from build123d import *

# Parameters (mm, degrees)
SKETCH_1_R      = 1.6
SKETCH_1_W      = 108
SKETCH_1_H      = 67.317279836
EXTRUDE_1_DEPTH = 2
FILLET_1_R      = 3


with BuildPart() as part:
    # ｽｹｯﾁ1 → ﾎﾞｽ - 押し出し1 (new body)
    with BuildSketch(Plane(origin=(0, 0, 0), x_dir=(1, 0, 0), z_dir=(0, 1, 0))):
        Polygon((-61, 40.658639918), (-135.317279836, 40.658639918), (-135.317279836, 60.658639918), (-142.317279836, 60.658639918), (-142.317279836, 40.658639918), (-61, -40.658639918), (61, -40.658639918), (142.317279836, 40.658639918), (142.317279836, 60.658639918), (135.317279836, 60.658639918), (135.317279836, 40.658639918), (61, 40.658639918), align=None)
        with Locations(Location((-57.5, -37.158639918, 0), (0, 0, 270))):
            Circle(SKETCH_1_R, mode=Mode.SUBTRACT)
        with Locations(Location((57.5, -37.158639918, 0), (0, 0, 270))):
            Circle(SKETCH_1_R, mode=Mode.SUBTRACT)
        with Locations(Location((-131.746212025, 37.087572106, 0), (0, 0, 270))):
            Circle(SKETCH_1_R, mode=Mode.SUBTRACT)
        with Locations(Location((131.746212025, 37.087572106, 0), (0, 0, 270))):
            Circle(SKETCH_1_R, mode=Mode.SUBTRACT)
        with Locations(Location((20, -37.158639918, 0), (0, 0, 270))):
            Circle(SKETCH_1_R, mode=Mode.SUBTRACT)
        with Locations(Location((-20, -37.158639918, 0), (0, 0, 270))):
            Circle(SKETCH_1_R, mode=Mode.SUBTRACT)
        with Locations(Location((20, 37.158639918, 0), (0, 0, 90))):
            Circle(SKETCH_1_R, mode=Mode.SUBTRACT)
        with Locations(Location((-20, 37.158639918, 0), (0, 0, 90))):
            Circle(SKETCH_1_R, mode=Mode.SUBTRACT)
        with Locations(Location((57.5, 37.158639918, 0), (0, 0, 270))):
            Circle(SKETCH_1_R, mode=Mode.SUBTRACT)
        with Locations(Location((57.5, -17.841360082, 0), (0, 0, 270))):
            Circle(SKETCH_1_R, mode=Mode.SUBTRACT)
        with Locations(Location((-57.5, -17.841360082, 0), (0, 0, 90))):
            Circle(SKETCH_1_R, mode=Mode.SUBTRACT)
        with Locations(Location((-57.5, 37.158639918, 0), (0, 0, 90))):
            Circle(SKETCH_1_R, mode=Mode.SUBTRACT)
        with Locations(Location((138.817279836, 55.658639918, 0), (0, 0, 270))):
            Circle(SKETCH_1_R, mode=Mode.SUBTRACT)
        with Locations(Location((138.817279836, 45.658639918, 0), (0, 0, 270))):
            Circle(SKETCH_1_R, mode=Mode.SUBTRACT)
        with Locations(Location((-138.817279836, 55.658639918, 0), (0, 0, 270))):
            Circle(SKETCH_1_R, mode=Mode.SUBTRACT)
        with Locations(Location((-138.817279836, 45.658639918, 0), (0, 0, 270))):
            Circle(SKETCH_1_R, mode=Mode.SUBTRACT)
        Rectangle(SKETCH_1_W, SKETCH_1_H, mode=Mode.SUBTRACT)
        Polygon((-125.4177849, 33.658639918), (-61, -30.759144982), (-61, 33.658639918), align=None, mode=Mode.SUBTRACT)
        Polygon((61, 33.658639918), (61, -30.759144982), (125.4177849, 33.658639918), align=None, mode=Mode.SUBTRACT)
    extrude(amount=EXTRUDE_1_DEPTH)

    # ﾌｨﾚｯﾄ1
    fillet_1_edges = [part.edges().sort_by_distance(p)[0] for p in [
        (135.317279836, 1, -40.658639918),
        (135.317279836, 1, -60.658639918),
        (142.317279836, 1, -60.658639918),
        (142.317279836, 1, -40.658639918),
        (61, 1, 40.658639918),
        (-61, 1, 40.658639918),
        (-142.317279836, 1, -40.658639918),
        (-142.317279836, 1, -60.658639918),
        (-135.317279836, 1, -60.658639918),
        (-135.317279836, 1, -40.658639918),
        (-54, 1, -33.658639918),
        (-54, 1, 33.658639918),
        (54, 1, 33.658639918),
        (54, 1, -33.658639918),
        (-61, 1, -33.658639918),
        (-125.4177849, 1, -33.658639918),
        (-61, 1, 30.759144982),
        (125.4177849, 1, -33.658639918),
        (61, 1, -33.658639918),
        (61, 1, 30.759144982),
    ]]
    fillet(fillet_1_edges, radius=FILLET_1_R)


solid = part.part
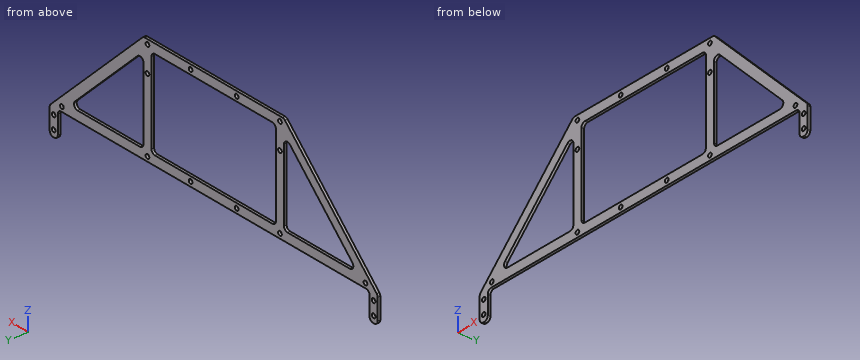
Read the model definition and answer for the solid it produces. Units are mm, in the model's axes. Give positions to 0.01 mm unless a question says otherwise; leave off trailing zeros. Write each loop counter-clockwise with the first axis right and the second up, starting at its lowest first coordinate (ties: lowest second). Pieces come first, ordered by that corner, then holes. Notation, with made-up numbers: (25.25, 23) - (72.25, 23) arc R16 cw to (72.25, 39) - close; hole circle Ø4 at (-15, -12.75). An arc over 180 degrees is marked (long way). Use CSV: the item, a comma, the result in double quotes. Start each with the question number.
Item 1: The part is cut by section D-D, the plane y = 0.4. Count the separate pieces of the cut face and the enclosed holes in it, and give its area (3 significant figures).
Item 2: Flat-ended cylindrical pins translate along their axes: P1, Ø2, axis at x = 93, z = -2.5, coming from the -Y side; P2, Ø0.6, axis at y = 0.5, z = 15, coming from the -X side; P3, Ø0.6, axis at x = 13.5, y = 0.5, coming from the -Z side. Find the tip coordinate at first contact, or state that the pin passes through.
Item 3: Consider line 1 (Z direction, x = 15, y = 1.2); line 2 (X direction, y = 1.15, z = 36.5); line 3 (X direction, y = 0.8, z = -45). Determine where each line is inside the solid, lowest interval first.
Item 4: The part is cut by section B-B, the plane z = -6. Give the vertices of the cut face in (x, y), and give its area (3 significant figures).
Item 5: The part is cut by section A-A, the plane x = -35.5. Give the vertices of the cut face in (y, z).
Item 6: The part is cut by section C-C, the plane x = -70. Give the vertices of the cut face in (y, z).
Taken from the geometry:
1,separate pieces,"1"
1,enclosed holes,"19"
1,area,"5,320 mm2"
2,P1,"y = 0"
2,P2,"x = -86.96"
2,P3,"z = -40.66"
3,line 1,"-40.66 to -33.66, 33.66 to 40.66"
3,line 2,"-65.16 to -58.96, -56.04 to -21.46, -18.54 to 18.54, 21.46 to 56.04, 58.96 to 65.16"
3,line 3,"-142.32 to -140.28, -137.36 to -135.32, 135.32 to 137.36, 140.28 to 142.32"
4,outline,"(-107.66, 0) - (-97.76, 0) - (-97.76, 2) - (-107.66, 2) - close; (-61, 0) - (-54, 0) - (-54, 2) - (-61, 2) - close; (54, 0) - (61, 0) - (61, 2) - (54, 2) - close; (97.76, 0) - (107.66, 0) - (107.66, 2) - (97.76, 2) - close"
4,area,"67.6 mm2"
5,outline,"(0, -40.66) - (2, -40.66) - (2, -33.66) - (0, -33.66) - close; (0, 33.66) - (2, 33.66) - (2, 40.66) - (0, 40.66) - close"
6,outline,"(0, -40.66) - (2, -40.66) - (2, -33.66) - (0, -33.66) - close; (0, 21.76) - (2, 21.76) - (2, 31.66) - (0, 31.66) - close"
